Design review of the part built by this model. Coordinates are the model's own, in mm. Coordinates: 2 decimals unless noted, no trailing zeros. Order: outer loops, then holes, each group sorted by start corner. A loop starts at its lowest first (then second) coordinate and runs counter-clockwise, first axis right, second up. Notation, with made-up numbers: M 20.5,78 L 53.5,78 A8 cw 53.5,91 Z; hole C 18.5,17 d8. An arc over 180 degrees is marked long. Answer in a Markdown table with one row per item.
from build123d import *

# Parameters (mm, degrees)
F0_R     = 20
F1_DEPTH = 20
F2_SIZE2 = 4.99999
F2_SIZE  = 19.99999
F3_R     = 19.6
F4_DEPTH = 19
F4_TAPER = 14


# Not quite as in the source:
# - a fillet or chamfer is up to 0.001 mm smaller than in the source, because OpenCascade refuses the exact size


with BuildPart() as f1:
    # F0 (on Top) → F1 (new body)
    with BuildSketch(Plane.XY):
        Circle(F0_R)
    extrude(amount=F1_DEPTH)

    # F2 (size 20 and 5 in the source; OpenCascade refuses exactly that, so slightly less here)
    f2_edges = [f1.edges().sort_by_distance(p)[0] for p in [
        (-20, 0, 0),
    ]]
    f2_side = f1.faces().sort_by_distance((-20, 0, 10))[0]
    chamfer(f2_edges, length=F2_SIZE, length2=F2_SIZE2, reference=f2_side)

    # F3 (on face) → F4 (cut)
    with BuildSketch(Plane.XY.offset(20)):
        Circle(F3_R)
    extrude(amount=-F4_DEPTH, taper=F4_TAPER, mode=Mode.SUBTRACT)


solid = f1.part
(1) For line 1 along X through (y, z) = (-11, 11.5); line 2 along Y through (x, z) = (2.5, 13.5); line 3 along Z through (x, y) = (0, -3), list the stretches that pass through material, from the lowest coordinate up. Write a range as from..to.
Return value:
| item | result |
|---|---|
| line 1 | x = -14.09..-13.59, 13.59..14.09 |
| line 2 | y = -18.2..-17.8, 17.8..18.2 |
| line 3 | z = 0..1 |
(2) Add section B-B, the plane z = 16. Give the boundary of the cut face in (x, y).
Return value:
| item | result |
|---|---|
| outline | C 0,0 d38; hole C 0,0 d37.21 |
(3) Draft analysis for pull direction Y (two halves, no side actions). For faces 1 (the conical face through (15.4, 4.85, 6.14)), 2 (the conical face through (-3.545, -15.965, 5.416)), 3 (the flat face through (13.2, -14.7, 20)), 4 (the flat face through (0, 0, 1)), state which applies: pulls with the +Y half, pulls with the -Y half, needs draft (parallel to the pull), parting line crosses it, or undercut.
Return value:
| item | result |
|---|---|
| face 1 | undercut |
| face 2 | parting line crosses it |
| face 3 | needs draft |
| face 4 | undercut |
(4) Insertion check: pin 1 Ø6 at (x, z) = (-2.5, 7) entering from +Y; pin 2 Ø8 at (x, z) = (8, 10) entering from -Y; pin 3 Ø1 at (y, z) = (8, 8.5) entering from -X. Each pin has a flat end and moves straight along its axis. Give the tip position at first contact, or say it passes through.
Return value:
| item | result |
|---|---|
| pin 1 | stops at y = 17.39 |
| pin 2 | stops at y = -17.46 |
| pin 3 | stops at x = -15.43 |
(5) Add section C-C, the plane z = 8.5. Give the boundary of the cut face in (x, y) (3 decimals), and give its area (3 significant figures).
Return value:
| item | result |
|---|---|
| outline | C 0,0 d34.25; hole C 0,0 d33.465 |
| area | 41.7 mm2 |
